Build history of the part. All positions in model axes, mm. A direction names the side the tool comes from. Round coordinates to 2 decimals unless told otherwise and drop trailing zeros. Write each loop counter-clockwise with the first axis right and the second up, starting at its lowest first coordinate (ties: lowest second). Pieces come first, ordered by that corner, then holes.
1) Saw through at B-B (x = -38.1). Write the cut outline in (y, z) (1 decimal), plus the area to 3 significant figures.
2) Saw through at D-D (x = 13.5). Write the cut outline in (y, z) (3 decimals), plus the area to 3 significant figures.
3) Wall check: probe 1 along X at (y, z) = (0.25, -165.1); probe 2 along Z at (x, y) = (-34.5, 0.25); probe 3 along X at (y, z) = (2, -129). Give the ranges that are in metal, low to high.
4) Pull direction X, two halves, no side cores. Call faces 1 (the flat face through (0, 0, 147)), 2 (the flat face through (-26, 0, 177.8)), 3 (the cylindrical face through (-37.891, -0.044, -160.342)): +X half, -X half, draft (parallel to the pull), parting line (faces both ways), or undercut.
5) Saw through at C-C (y = -0.5). Write the cut outline in (x, z) (1 decimal).
6) Which spindle directions (+Z, -Z, +X, -X, +Y, -Y) get a long thin tool onto all of the face, cutting with end or side? Do faces 4 (the flat face through (19, 0, 117.475)), 5 (the flat face through (38.1, 0, 2)), 6 (the flat face through (19, 0, -117.475)). Say none if no direction does.
7) Saw through at A-A (z = -165.1). Write the cut outline in (x, y) (1 decimal), plus the area to 3 significant figures.
8) Flat gauge pins, fed straight in: pin 1 (1.9 mm diameter, centred on x = 25.5, y = 1.5, fed in from +Z) (3 decimals); pin 2 (5.5 mm diameter, centred on x = -38.1, z = 165.1, fed in from -Y); pin 3 (3 mm diameter, centred on x = 16, y = 1, fed in from -Z) (3 decimals); pin 4 (3 mm diameter, centred on y = -1.5, z = 152.5, fed in from +X). Where does each tip first touch, or does it go through?
from build123d import *

# Parameters (mm, degrees)
SKETCH1_W                   = 165.1
SKETCH1_H                   = 38.1
BOSS_EXTRUDE1_DEPTH         = 3.175
F_1_4_0_25_DIAMETER_HOLE1_D = 7.9375
SKETCH4_W                   = 50.8
SKETCH4_H                   = 355.6
SKETCH4_R                   = 4.7625
BOSS_EXTRUDE2_DEPTH         = 6.35
SKETCH5_W                   = 165.1
SKETCH5_H                   = 76.2
CUT_EXTRUDE1_DEPTH          = 271.08036304
SKETCH6_W                   = 38.1
SKETCH6_H                   = 60.325
CUT_EXTRUDE2_DEPTH          = 186.023789011


with BuildPart() as part:
    # Sketch1 → Boss-Extrude1 (new, symmetric)
    with BuildSketch(Plane(origin=(0, 0, 0), x_dir=(1, 0, 0), z_dir=(0, 1, 0))):
        Polygon((0, 0), (0, -177.8), (38.1, -177.8), (38.1, -38.1), (38.1, 0), align=None)
        with Locations((120.65, -19.05)):
            Rectangle(SKETCH1_W, SKETCH1_H)
        with Locations((120.65, 19.05)):
            Rectangle(SKETCH1_W, SKETCH1_H)
        Polygon((0, 177.8), (0, 0), (38.1, 0), (38.1, 38.1), (38.1, 177.8), align=None)
    extrude(amount=BOSS_EXTRUDE1_DEPTH, both=True)

    # 1/4 (0.25) Diameter Hole1 (through all)
    with Locations(Plane(origin=(0, 3.175, 0), x_dir=(1, 0, 0), z_dir=(0, 1, 0))):
        with Locations((190.5, 25.4), (190.5, -25.4)):
            Hole(F_1_4_0_25_DIAMETER_HOLE1_D / 2)

    # Sketch4 → Boss-Extrude2 (add)
    with BuildSketch(Plane.XZ.offset(3.175)):
        with Locations((-25.4, 0)):
            Rectangle(SKETCH4_W, SKETCH4_H)
        with Locations(Location((-38.1, -165.1, 0), (0, 0, 270))):
            Circle(SKETCH4_R, mode=Mode.SUBTRACT)
        with Locations(Location((-38.1, 165.1, 0), (0, 0, 270))):
            Circle(SKETCH4_R, mode=Mode.SUBTRACT)
    extrude(amount=-BOSS_EXTRUDE2_DEPTH)

    # Sketch5 → Cut-Extrude1 (cut, through all)
    with BuildSketch(Plane.XZ.offset(3.175)):
        with Locations((120.65, 0)):
            Rectangle(SKETCH5_W, SKETCH5_H)
    extrude(amount=-CUT_EXTRUDE1_DEPTH, mode=Mode.SUBTRACT)

    # Sketch6 → Cut-Extrude2 (cut, through all)
    with BuildSketch(Plane.XZ.offset(3.175)):
        with Locations((19.05, 147.6375)):
            Rectangle(SKETCH6_W, SKETCH6_H)
        with Locations((19.05, -147.6375)):
            Rectangle(SKETCH6_W, SKETCH6_H)
    extrude(amount=-CUT_EXTRUDE2_DEPTH, mode=Mode.SUBTRACT)


solid = part.part
Evaluation:
1. outline: (-3.2, -177.8) - (3.2, -177.8) - (3.2, -169.9) - (-3.2, -169.9) - close; (-3.2, -160.3) - (3.2, -160.3) - (3.2, 160.3) - (-3.2, 160.3) - close; (-3.2, 169.9) - (3.2, 169.9) - (3.2, 177.8) - (-3.2, 177.8) - close
1. area: 2,140 mm2
2. outline: (-3.175, -117.475) - (3.175, -117.475) - (3.175, 117.475) - (-3.175, 117.475) - close
2. area: 1,490 mm2
3. probe 1: x = -50.8 to -42.86, -33.34 to 0
3. probe 2: z = -177.8 to -168.22, -161.98 to 161.98, 168.22 to 177.8
3. probe 3: x = -50.8 to 0
4. face 1: +X half
4. face 2: draft
4. face 3: undercut
5. outline: (-50.8, -177.8) - (0, -177.8) - (0, -117.5) - (38.1, -117.5) - (38.1, 117.5) - (0, 117.5) - (0, 177.8) - (-50.8, 177.8) - close; hole circle Ø9.5 at (-38.1, -165.1); hole circle Ø9.5 at (-38.1, 165.1)
6. face 4: +Z, +X, +Y, -Y
6. face 5: +Z, -Z, +X, +Y, -Y
6. face 6: -Z, +X, +Y, -Y
7. outline: (-50.8, -3.2) - (-42.9, -3.2) - (-42.9, 3.2) - (-50.8, 3.2) - close; (-33.3, -3.2) - (0, -3.2) - (0, 3.2) - (-33.3, 3.2) - close
7. area: 262 mm2
8. pin 1: stops at z = 117.475
8. pin 2: passes through
8. pin 3: stops at z = -117.475
8. pin 4: stops at x = 0
